Geometry: final body of the model. Coordinates: model frame, mm. Face numbers are marked on the shaded views. Coordinates: 2 decimals unless noted, no trailing zeros. Write each loop counter-clockwise with the first axis right and the second up, starting at its lowest first coordinate (ties: lowest second). Pieces come first, ordered by that corner, then holes.
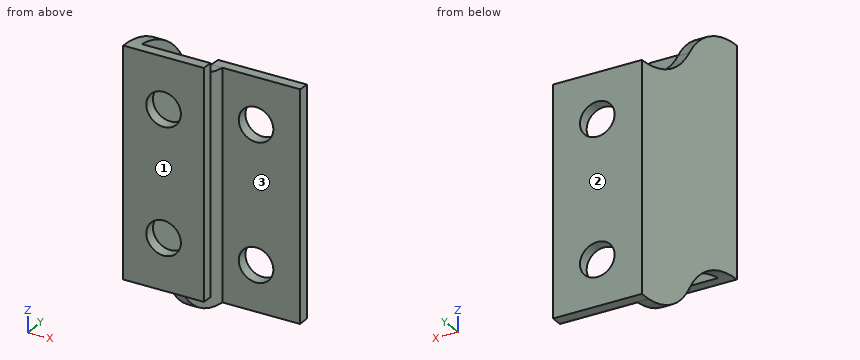
from build123d import *

# Parameters (mm, degrees)
BOSS_EXTRUDE1_DEPTH = 28.5
SKETCH5_R           = 1.5
CUT_EXTRUDE4_DEPTH  = 1
SKETCH11_W          = 1
SKETCH11_H          = 12.5
CUT_EXTRUDE5_DEPTH  = 10
SKETCH12_W          = 20.843481987
SKETCH12_H          = 1.334220042
CUT_EXTRUDE7_DEPTH  = 1
SKETCH13_R          = 1.5
CUT_EXTRUDE8_DEPTH  = 1


with BuildPart() as part:
    # Sketch1 → Boss-Extrude1 (new body)
    with BuildSketch(Plane.XY):
        Polygon((397.82422908, 16), (397.423944987, 2.5), (405.423944987, 2.5), (405.423944987, 3.5), (398.454035145, 3.5), (398.795017891, 15), (405.52422908, 15), (405.52422908, 16), align=None)
    extrude(amount=BOSS_EXTRUDE1_DEPTH)

    # Sketch5 → Cut-Extrude4 (cut)
    with BuildSketch(Plane(origin=(0, 16, 0), x_dir=(1, 0, 0), z_dir=(0, 1, 0))):
        with Locations(Location((401.703493459, -5, 0), (0, 0, 270))):
            Circle(SKETCH5_R)
        with Locations(Location((401.703493459, -17, 0), (0, 0, 270))):
            Circle(SKETCH5_R)
    extrude(amount=-CUT_EXTRUDE4_DEPTH, mode=Mode.SUBTRACT)

    # Sketch11 → Cut-Extrude5 (cut)
    with BuildSketch(Plane(origin=(405.52422908, 0, 0), x_dir=(0, 0, -1), z_dir=(1, 0, 0))):
        with BuildLine():
            ThreePointArc((-24.75, 9.25), (-22.257567862, 11.708863545), (-21.063143846, 15))
            Line((-21.063143846, 15), (-28.5, 15))
            Line((-28.5, 15), (-28.5, 2.5))
            ThreePointArc((-28.5, 2.5), (-27.499550345, 6.360861303), (-24.75, 9.25))
        make_face()
        with BuildLine():
            ThreePointArc((-21.063143846, 15), (-21.015801665, 15.499004205), (-21, 16))
            Line((-21, 16), (-28.5, 16))
            Line((-28.5, 16), (-28.5, 15))
            Line((-28.5, 15), (-21.063143846, 15))
        make_face()
        with Locations((-0.5, 8.75)):
            Rectangle(SKETCH11_W, SKETCH11_H)
        with BuildLine():
            Line((0, 15), (0, 16))
            Line((0, 16), (-1, 16))
            ThreePointArc((-1, 16), (-0.986298018, 15.553268089), (-1, 15.106536177))
            Line((-1, 15.106536177), (-1, 15))
            Line((-1, 15), (0, 15))
        make_face()
        with BuildLine():
            Line((-1, 2.5), (-1, 15))
            Line((-1, 15), (-1.007325107, 15))
            ThreePointArc((-1.007325107, 15), (-2.100816605, 11.679499144), (-4.614575443, 9.25))
            ThreePointArc((-4.614575443, 9.25), (-7.459265697, 6.394195167), (-8.5, 2.5))
            Line((-8.5, 2.5), (-2.5, 2.5))
            Line((-2.5, 2.5), (-1, 2.5))
        make_face()
    extrude(amount=-CUT_EXTRUDE5_DEPTH, mode=Mode.SUBTRACT)

    # Sketch12 → Cut-Extrude7 (cut)
    with BuildSketch(Plane(origin=(405.423944987, 0, 0), x_dir=(0, 0, -1), z_dir=(1, 0, 0))):
        with Locations((-18.404841791, 2.845743799)):
            Rectangle(SKETCH12_W, SKETCH12_H)
    extrude(amount=-CUT_EXTRUDE7_DEPTH, mode=Mode.SUBTRACT)

    # Sketch13 → Cut-Extrude8 (cut)
    with BuildSketch(Plane.XZ.offset(-2.5)):
        with Locations((400.923944987, 24)):
            Circle(SKETCH13_R)
        with Locations((400.923944987, 13)):
            Circle(SKETCH13_R)
    extrude(amount=-CUT_EXTRUDE8_DEPTH, mode=Mode.SUBTRACT)


solid = part.part
Item 1: Section C-C, the plane x = 405.25. Output: boundary loops of the cut face in (y, z), plus the area to 3 significant figures.
Derived:
outline: (15, 1) - (15.11, 1) arc R7.29 ccw to (16, 1) - (16, 21) arc R7.95 cw to (15, 21.06) - close
area: 20.0 mm2
Item 2: Material intervals for probe 1 along Y at (x, z) = (404.25, 11.75); probe 2 along Y at (x, z) = (401.25, 12.75); probe 3 along X at (y, z) = (15.7, 5), sorted ascending.
Derived:
probe 1: y = 2.5 to 3.5, 15 to 16
probe 2: y = 15 to 16
probe 3: x = 397.82 to 400.2, 403.2 to 405.52
Item 3: Pull-direction query (Y, two-part tool) for the marked faces 1, 2 and 3; classes: released by +Y, released by -Y, zero draft, split by the parting line, or undercut.
Derived:
face 1: released by -Y
face 2: released by +Y
face 3: undercut
Item 4: Pin query (flat end, axial travel): pin 1 (2.5 mm diameter, centred on x = 400.92, z = 13, fed in from -Y); pin 2 (4 mm diameter, centred on y = 8.5, z = 9, fed in from -X). Return the tip coordinate at first contact, or that it passes through.
Derived:
pin 1: stops at y = 15
pin 2: stops at x = 397.54
Item 5: Section A-A, the plane x = 403.75. Output: boundary loops of the cut face in (y, z).
Derived:
outline: (2.5, 8.5) arc R7.81 cw to (3.5, 8.44) - (3.5, 28.44) arc R7.95 ccw to (2.5, 28.5) - close; (15, 1) - (15.11, 1) arc R7.29 ccw to (16, 1) - (16, 21) arc R7.95 cw to (15, 21.06) - close
Item 6: Section D-D, the plane z = 24. Output: boundary loops of the cut face in (x, y).
Derived:
outline: (397.42, 2.5) - (399.42, 2.5) - (399.42, 3.5) - (398.45, 3.5) - (398.64, 9.78) - (397.64, 9.78) - close; (402.42, 2.5) - (404.42, 2.5) - (404.42, 3.5) - (402.42, 3.5) - close
Item 7: Section B-B, the plane z = 17. Output: boundary loops of the cut face in (x, y).
Derived:
outline: (397.42, 2.5) - (404.42, 2.5) - (404.42, 3.5) - (398.45, 3.5) - (398.8, 15) - (400.2, 15) - (400.2, 16) - (397.82, 16) - close; (403.2, 15) - (405.52, 15) - (405.52, 16) - (403.2, 16) - close
